from build123d import *

# Parameters (mm, degrees)
SKETCH1_R           = 11
BOSS_EXTRUDE1_DEPTH = 47.2
SKETCH2_R           = 5
BOSS_EXTRUDE2_DEPTH = 1
SKETCH3_R           = 1.5
BOSS_EXTRUDE3_DEPTH = 10
SKETCH4_R           = 1
CUT_EXTRUDE1_DEPTH  = 2.5


with BuildPart() as part:
    # Sketch1 → Boss-Extrude1 (new body)
    with BuildSketch(Plane.XY):
        Circle(SKETCH1_R)
    extrude(amount=-BOSS_EXTRUDE1_DEPTH)

    # Sketch2 → Boss-Extrude2 (add)
    with BuildSketch(Plane.XY):
        Circle(SKETCH2_R)
    extrude(amount=BOSS_EXTRUDE2_DEPTH)

    # Sketch3 → Boss-Extrude3 (add)
    with BuildSketch(Plane.XY):
        Circle(SKETCH3_R)
    extrude(amount=BOSS_EXTRUDE3_DEPTH)

    # Sketch4 → Cut-Extrude1 (cut)
    with BuildSketch(Plane.XY):
        with Locations((0, 8.5)):
            Circle(SKETCH4_R)
        with Locations((7.361215932, -4.25)):
            Circle(SKETCH4_R)
        with Locations((-7.361215932, -4.25)):
            Circle(SKETCH4_R)
    extrude(amount=-CUT_EXTRUDE1_DEPTH, mode=Mode.SUBTRACT)


solid = part.part
Here's how the part is built. I have some questions about the finished solid (model axes, mm). A direction names the side the tool comes from. Coordinates: 2 decimals unless noted, no trailing zeros. Loops run counter-clockwise (first coordinate to the right, second up) from the corner with the lowest first, then second, coordinate; pieces in that order, holes last.
1. Imagine slicing it at B-B, the plane y = 0. Please give me the cut outline in (x, z).
2. I need wall thicknesses on L1, parallel to Y at x = 0, z = -1.45; L2, parallel to Z at x = 6.5, y = -8; L3, parallel to Y at x = 0.25, z = -24.5. Which ranges of each line are inside material? Lowest first, please.
3. If we mould it in two halves opening along X, with no side actions, what happens to faces 1 (the flat face through (-1.2, 1.2, 1)), 2 (the flat face through (0, 9, -2.5)), 3 (the cylindrical face through (-2.38, -10.74, -23.27))? For each: pulls with the +X half, pulls with the -X half, needs draft (parallel to the pull), parting line crosses it, or undercut.
4. Imagine slicing it at D-D, the plane x = -3. Please give me the cut outline in (y, z).
5. Imagine slicing it at C-C, the plane z = -42. Please give me the cut outline in (x, y), and give its area (3 significant figures).
6. For P1, Ø1, axis at x = -5.5, z = -40.5, coming from the -Y side; P2, Ø5, axis at x = -6, z = -33, coming from the +Y side; P3, Ø1, axis at y = 5, z = -2.5, coming from the -X side; P4, Ø2, axis at x = -9, y = 8, coming from the +Z side, each with a flat end and sliding along its axis, tell me the tip position at first contact or that it passes through.
7. Imagine slicing it at A-A, the plane x = 0. Please give me the cut outline in (y, z), and give its area (3 significant figures).
8. For faces 4 (the flat face through (0, 0, 10)), 5 (the cylindrical face through (-8.098, -3.574, -1.232)), which set-ups out of +Z, -Z, +X, -X, +Y, -Y let a thin tool reach every point of the face, with its end or its side?
Taken from the geometry:
1. outline: (-11, -47.2) - (11, -47.2) - (11, 0) - (5, 0) - (5, 1) - (1.5, 1) - (1.5, 10) - (-1.5, 10) - (-1.5, 1) - (-5, 1) - (-5, 0) - (-11, 0) - close
2. L1: y = -11 to 7.5, 9.5 to 11
2. L2: z = -47.2 to 0
2. L3: y = -11 to 11
3. face 1: needs draft
3. face 2: undercut
3. face 3: parting line crosses it
4. outline: (-10.58, -47.2) - (10.58, -47.2) - (10.58, 0) - (4, 0) - (4, 1) - (-4, 1) - (-4, 0) - (-10.58, 0) - close
5. outline: circle Ø22 at (0, 0)
5. area: 380 mm2
6. P1: stops at y = -9.8
6. P2: stops at y = 10.43
6. P3: stops at x = -10.04
6. P4: passes through
7. outline: (-11, -47.2) - (11, -47.2) - (11, 0) - (9.5, 0) - (9.5, -2.5) - (7.5, -2.5) - (7.5, 0) - (5, 0) - (5, 1) - (1.5, 1) - (1.5, 10) - (-1.5, 10) - (-1.5, 1) - (-5, 1) - (-5, 0) - (-11, 0) - close
7. area: 1,070 mm2
8. face 4: +Z, +X, -X, +Y, -Y
8. face 5: +Z
